Source: CAD feature listing. Evaluate the final solid. Frame: model axes, mm. A direction names the side the tool comes from. Give positions to 0.01 mm unless a question says otherwise; leave off trailing zeros. Write each loop counter-clockwise with the first axis right and the second up, starting at its lowest first coordinate (ties: lowest second). Pieces come first, ordered by that corner, then holes. Notation, with made-up numbers: (89.5, -17) -> (135.5, -17) arc R20 ccw to (135.5, -10) -> close; hole circle Ø8 at (-13.5, 7.5). An arc over 180 degrees is marked (long way). Use one line per item in the form item = value. Start each with the question number.
(1) Cut plane A-A, the plane y = 0. Output: boundary loops of the cut face in (x, z).
(2) First-contact query: P1, Ø14.5, axis at y = 7, z = -1, coming from the -X side; P2, Ø5, axis at x = -3, z = -3.5, coming from the +Y side; P3, Ø4, axis at y = 0, z = 8.5, coming from the +X side. Flat tips, straight axial feed; report the tip coordinate or a pass-through.
(3) Cut plane C-C, the plane x = -6.75. Output: boundary loops of the cut face in (y, z), and give its area (3 significant figures).
(4) Material intervals for line 1 along Z through (x, y) = (-3.2, 0); line 2 along Z through (x, y) = (-8.05, 0), sorted ascending. Write a range as from..to.
(5) Cut plane D-D, the plane x = -3.75. Output: boundary loops of the cut face in (y, z).
(6) Draft query along Z for faces 4 (the face through (-17, -1, -15)), 5 (the face through (-7, 1.118, 0)), 6 (the face through (-8.42, 20.03, -6.31)). Return one class per face: pulls with the +Z half, pulls with the -Z half, needs draft (parallel to the pull), parting line crosses it, or undercut.
(7) Cut plane B-B, the plane z = 0. Output: boundary loops of the cut face in (x, y), and give its area (3 significant figures).
(8) Set-up query: faces 1 (the face through (-13.056, 6.691, 12.864)), 2 (the face through (-5, 3, 0)), 3 (the face through (0, 1, -15)). Return all of +Z, -Z, +X, -X, +Y, -Y with unobstructed straight access to the full face (end or side cutting, diameter ignored); none if empty.
from build123d import *

# Parameters (mm, degrees)
CONG_1_R                = 3
ENL_V_MAT_EXTRU_1_REACH = 34.031


with BuildPart() as part:
    # Esquisse1 → Révolution1 (revolve)
    with BuildSketch(Plane.XY):
        Polygon((-17, 21), (0, 21), (0, 14.5), (-5, 14.5), (-5, 0), (-9, 0), (-9, 14.5), (-17, 14.5), align=None)
    revolve(axis=Axis((-5, 0, 0), (-1, 0, 0)))

    # Congé1
    cong_1_edges = [part.edges().sort_by_distance(p)[0] for p in [
        (-17, -21, 0),
        (0, -21, 0),
    ]]
    fillet(cong_1_edges, radius=CONG_1_R)

    # Esquisse2 → Enlèv. mat.-Extru.1 (cut, up to next)
    with BuildSketch(Plane(origin=(-5, 0, 0), x_dir=(0, 0, -1), z_dir=(1, 0, 0)), mode=Mode.PRIVATE) as enl_v_mat_extru_1_sk1:
        with BuildLine():
            Line((-1, 1.118033989), (1, 1.118033989))
            ThreePointArc((1, 1.118033989), (0, -1.5), (-1, 1.118033989))
        make_face()
    enl_v_mat_extru_1_tool1 = extrude(enl_v_mat_extru_1_sk1.sketch, amount=-ENL_V_MAT_EXTRU_1_REACH, mode=Mode.PRIVATE) & part.part
    add(enl_v_mat_extru_1_tool1.solids().sort_by_distance((-5, -0.101863, 0))[0], mode=Mode.SUBTRACT)


solid = part.part
Geometry says:
q1.outline = (-17, -18) arc R3 ccw to (-14, -21) -> (-3, -21) arc R3 ccw to (0, -18) -> (0, -14.5) -> (-5, -14.5) -> (-5, -1.5) -> (-9, -1.5) -> (-9, -14.5) -> (-17, -14.5) -> close; (-17, 14.5) -> (-9, 14.5) -> (-9, 1.5) -> (-5, 1.5) -> (-5, 14.5) -> (0, 14.5) -> (0, 18) arc R3 ccw to (-3, 21) -> (-14, 21) arc R3 ccw to (-17, 18) -> close
q2.P1 = -9
q2.P2 = 20.98
q2.P3 = -5
q3.outline = circle Ø42 at (0, 0); hole (1.12, -1) -> (1.12, 1) arc R1.5 ccw (long way) to start
q3.area = 1,380 mm^2
q4.line_1 = -21..-14.5, 14.5..21
q4.line_2 = -21..-1.5, 1.5..21
q5.outline = circle Ø42 at (0, 0); hole circle Ø29 at (0, 0)
q6.face_4 = needs draft
q6.face_5 = undercut
q6.face_6 = parting line crosses it
q7.outline = (-17, -18) arc R3 ccw to (-14, -21) -> (-3, -21) arc R3 ccw to (0, -18) -> (0, -14.5) -> (-5, -14.5) -> (-5, -1.5) -> (-9, -1.5) -> (-9, -14.5) -> (-17, -14.5) -> close; (-17, 14.5) -> (-9, 14.5) -> (-9, 1.12) -> (-5, 1.12) -> (-5, 14.5) -> (0, 14.5) -> (0, 18) arc R3 ccw to (-3, 21) -> (-14, 21) arc R3 ccw to (-17, 18) -> close
q7.area = 319 mm^2
q8.face_1 = -X
q8.face_2 = +X
q8.face_3 = +Z, -Z, +X, +Y, -Y
